from build123d import *

# Parameters (mm, degrees)
F0_R          = 12.7
F0_R_2        = 6.35
F1_DEPTH      = 0.9525
F2_DEPTH      = 7.3025
F2_DEPTH_BACK = 0.9525
F3_R          = 1.651
F4_DEPTH      = 8.255


with BuildPart() as f1:
    # F0 (on Front) → F1 (new body, symmetric)
    with BuildSketch(Plane.XZ):
        Circle(F0_R)
        Circle(F0_R_2, mode=Mode.SUBTRACT)
    extrude(amount=F1_DEPTH, both=True)

    # F0 (on Front) → F2 (join, two sides)
    with BuildSketch(Plane.XZ) as f2_sk:
        Circle(F0_R_2)
        with BuildLine():
            ThreePointArc((-1.09601, -1.0240908553), (0, 1.5), (1.09601, -1.0240908553))
            Line((1.09601, -1.0240908553), (-1.09601, -1.0240908553))
        make_face(mode=Mode.SUBTRACT)
    extrude(amount=-F2_DEPTH)
    extrude(f2_sk.sketch, amount=F2_DEPTH_BACK)

    # F3 (on face) → F4 (join)
    with BuildSketch(Plane.XZ.offset(0.9525)):
        with Locations((0, 10.0402068998)):
            Circle(F3_R)
        with Locations((7.063929059, 7.1827068998)):
            Circle(F3_R)
        with Locations((7.3034819544, -7.1827068998)):
            Circle(F3_R)
        with Locations((0, -10.2797931002)):
            Circle(F3_R)
        with Locations((10.1592937556, 0)):
            Circle(F3_R)
        with Locations((-7.1837055067, 7.0649111522)):
            Circle(F3_R)
        with Locations((-10.1592937556, 0)):
            Circle(F3_R)
        with Locations((-7.1837055067, -7.3044973525)):
            Circle(F3_R)
    extrude(amount=-F4_DEPTH)


solid = f1.part
Input: part model. Units: mm. Frame: model coordinates. A direction names the side the tool comes from. Coordinates: 2 decimals unless noted, no trailing zeros. Order: outer loops, then holes, each group sorted by start corner. A loop starts at its lowest first (then second) coordinate and runs counter-clockwise, first axis right, second up.
1. Cut plane A-A, the plane x = 0. Return loops of the section in (y, z), plus the area to 3 significant figures.
Checked values:
outline: (-0.95, -12.7) - (0.95, -12.7) - (0.95, -11.93) - (7.3, -11.93) - (7.3, -8.63) - (0.95, -8.63) - (0.95, -6.35) - (7.3, -6.35) - (7.3, -1.02) - (-0.95, -1.02) - close; (-0.95, 1.5) - (7.3, 1.5) - (7.3, 6.35) - (0.95, 6.35) - (0.95, 8.39) - (7.3, 8.39) - (7.3, 11.69) - (0.95, 11.69) - (0.95, 12.7) - (-0.95, 12.7) - close
area: 150 mm2
2. Cut plane D-D, the plane y = 0.25. Return loops of the section in (x, z), plus the area to 3 significant figures.
Checked values:
outline: circle Ø25.4 at (0, 0); hole (-1.1, -1.02) - (1.1, -1.02) arc R1.5 ccw (long way) to start
area: 500 mm2
3. Access query for faces 4 (the flat face through (0, 3, -1.024)), 5 (the flat face through (-7, 7.303, -7)), 6 (the cylindrical face through (-1.38, 4.08, -6.2)). Directions: +Z, -Z, +X, -X, +Y, -Y. A direction counts if a zero-diameter tool reaches every point of the face in a straight line with its end or side. Return the directions, or none.
Checked values:
face 4: +Y, -Y
face 5: +Z, -Z, +X, -X, +Y
face 6: +Y
4. Ray query, line 1 along Z through (x, y) = (0, 5.5); line 2 along Z through (x, y) = (-1.25, 1.25); line 3 along Y through (x, z) = (9.25, 4). Return the intervals inside material, ascending.
Checked values:
line 1: z = -11.93 to -8.63, -6.35 to -1.02, 1.5 to 6.35, 8.39 to 11.69
line 2: z = -11.36 to -9.2, -6.23 to -0.83, 0.83 to 6.23, 8.96 to 11.12
line 3: y = -0.95 to 0.95
5. Contact query for flat-ended pins moving along their axis: P1, Ø3, axis at y = 3.5, z = 1.5, coming from the +X side; P2, Ø1.5, axis at x = -5.5, y = 3, coming from the +Z side; P3, Ø1, axis at x = 3.5, y = 0.5, coming from the -Z side. Output: stop coordinate, or through.
Checked values:
P1: stops at x = 11.81
P2: stops at z = 8.43
P3: stops at z = -12.34
6. Draft query along X for faces 1 (the flat face through (0, 7.303, -10)), 2 (the cylindrical face through (-2.75, -0.01, -12.4)), 3 (the cylindrical face through (-8.833, 4.083, -7.232)). Return one class per face: +X half, -X half, draft (parallel to the pull), parting line (faces both ways), or undercut.
Checked values:
face 1: draft
face 2: parting line
face 3: undercut
7. Cut plane B-B, the plane z = 0. Return loops of the section in (x, y).
Checked values:
outline: (-12.7, -0.95) - (-1.5, -0.95) - (-1.5, 7.3) - (-6.35, 7.3) - (-6.35, 0.95) - (-8.51, 0.95) - (-8.51, 7.3) - (-11.81, 7.3) - (-11.81, 0.95) - (-12.7, 0.95) - close; (1.5, -0.95) - (12.7, -0.95) - (12.7, 0.95) - (11.81, 0.95) - (11.81, 7.3) - (8.51, 7.3) - (8.51, 0.95) - (6.35, 0.95) - (6.35, 7.3) - (1.5, 7.3) - close
8. Cut plane C-C, the plane y = 6.25. Count the separate pieces of the cut face and the enclosed holes in it, plus the area to 3 significant figures.
Checked values:
separate pieces: 9
enclosed holes: 1
area: 189 mm2
